Can you work these out from the model? Positions are in its coordinate system, mm. Give positions to 0.01 mm unless a question says otherwise; leave off trailing zeros.
1. I'm going to push flat-ended pins straight in: pin 1 (0.9 mm diameter, centred on y = -2.5, z = 22, fed in from -X); pin 2 (0.9 mm diameter, centred on y = -5, z = 22.5, fed in from +X). Where does each tip first touch, or does it pass through?
2. Suppose I cut it at A-A (x = 1.5). Give the number of separate pieces and of enclosed holes in the cut face, and give its area (3 significant figures).
3. If I drill on probe 1 along X at (y, z) = (-7, 5.5); probe 2 along X at (y, z) = (-7.25, -21); probe 3 along X at (y, z) = (-4.75, 10.5), over which ranges is the centre line in solid material (lowest first)?
```python
from build123d import *

# Parameters (mm, degrees)
F1_DEPTH = 10
F2_W     = 30
F2_H     = 3
F2_W_2   = 60
F3_DEPTH = 25
F4_W     = 30
F4_H     = 3
F4_W_2   = 60
F5_DEPTH = 25


with BuildPart() as f1:
    # F0 (on Front) → F1 (new body)
    with BuildSketch(Plane.XZ):
        Polygon((-40, -40), (0, -40), (0, -37), (-30.663718, -37), (-30.663718, -34), (0, -34), (0, -22), (-30.663718, -22), (-30.663718, -19), (-21.106195, -19), (-20.50885, -19), (0, -19), (0, -10), (-30.663718, -10), (-30.663718, -7), (0, -7), (0, 50), (-40, 50), (-40, -13), (-10, -13), (-10, -16), (-20.50885, -16), (-21.106195, -16), (-40, -16), (-40, -28), (-10, -28), (-10, -31), (-40, -31), align=None)
        Polygon((0, -40), (40, -40), (40, -31), (10, -31), (10, -28), (40, -28), (40, -16), (10, -16), (10, -13), (40, -13), (40, 50), (0, 50), (0, -7), (29.336282, -7), (29.336282, -10), (0, -10), (0, -19), (29.336282, -19), (29.336282, -22), (0, -22), (0, -34), (29.336282, -34), (29.336282, -37), (0, -37), align=None)
    extrude(amount=F1_DEPTH)

    # F2 (on face) → F3 (cut)
    with BuildSketch(Plane.XZ.offset(10)):
        with Locations((-25, -1.5)):
            Rectangle(F2_W, F2_H)
        with Locations((25, -1.5)):
            Rectangle(F2_W, F2_H)
        with Locations((-0.789474, 4.5)):
            Rectangle(F2_W_2, F2_H)
        with Locations((-25, 10.5)):
            Rectangle(F2_W, F2_H)
        with Locations((25, 10.5)):
            Rectangle(F2_W, F2_H)
        with Locations((1.97369, 16.5)):
            Rectangle(F2_W_2, F2_H)
        with Locations((-25, 22.5)):
            Rectangle(F2_W, F2_H)
        with Locations((25, 22.5)):
            Rectangle(F2_W, F2_H)
        with Locations((-0.789474, 28.5)):
            Rectangle(F2_W_2, F2_H)
    extrude(amount=-F3_DEPTH, mode=Mode.SUBTRACT)

    # F4 (on face) → F5 (cut)
    with BuildSketch(Plane.XZ.offset(10)):
        with Locations((-25, 35.5)):
            Rectangle(F4_W, F4_H)
        with Locations((25, 35.5)):
            Rectangle(F4_W, F4_H)
        with Locations((-1.184211, 41.5)):
            Rectangle(F4_W_2, F4_H)
        with Locations((-25, 47.5)):
            Rectangle(F4_W, F4_H)
        with Locations((25, 47.5)):
            Rectangle(F4_W, F4_H)
    extrude(amount=-F5_DEPTH, mode=Mode.SUBTRACT)


solid = f1.part
```
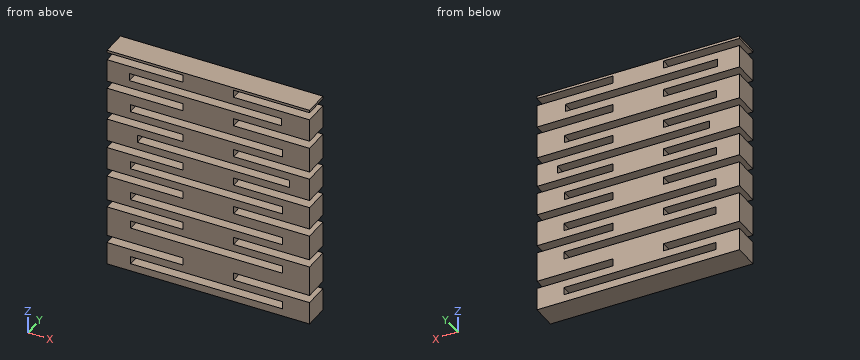
Checks:
1. pin 1: stops at x = -10
1. pin 2: stops at x = 10
2. separate pieces: 8
2. enclosed holes: 0
2. area: 690 mm2
3. probe 1: x = -40 to -30.79, 29.21 to 40
3. probe 2: x = -40 to -30.66, 29.34 to 40
3. probe 3: x = -10 to 10
